```python
from build123d import *

# Parameters (mm, degrees)
F1_DEPTH = 26
F2_R     = 1
F3_SIZE  = 1
F5_DEPTH = 6.5


with BuildPart() as f1:
    # F0 (on Front) → F1 (new body)
    with BuildSketch(Plane.XZ):
        Polygon((-27.5, -55), (-20.5, -55), (27.5, -36.5), (27.5, -26.5), (-17.5, -26.5), (-17.5, 26.5), (27.5, 26.5), (27.5, 36.5), (-20.5, 55), (-27.5, 55), (-27.5, 22.5), (-24, 22.5), (-24, -22.5), (-27.5, -22.5), align=None)
        Polygon((-20.5, -31.5), (26.5698068675, -31.5), (-20.5, -49.6414880635), align=None, mode=Mode.SUBTRACT)
        Polygon((-20.5, 31.5), (-20.5, 49.6414880635), (26.5698068675, 31.5), align=None, mode=Mode.SUBTRACT)
    extrude(amount=F1_DEPTH)

    # F2
    f2_edges = [f1.edges().sort_by_distance(p)[0] for p in [
        (-20.5, -13, 49.641488),
        (-20.5, -13, 31.5),
        (26.569807, -13, 31.5),
        (26.569807, -13, -31.5),
        (-20.5, -13, -31.5),
        (-20.5, -13, -49.641488),
        (-24, -13, -22.5),
        (-24, -13, 22.5),
    ]]
    fillet(f2_edges, radius=F2_R)

    # F3
    f3_edges = [f1.edges().sort_by_distance(p)[0] for p in [
        (27.5, -13, -26.5),
        (27.5, -13, 26.5),
    ]]
    chamfer(f3_edges, length=F3_SIZE)

    # F4 (on face) → F5 (cut, through all)
    with BuildSketch(Plane.YZ.offset(-17.5)):
        with BuildLine():
            ThreePointArc((-9.25, 8), (-9.8357864376, 9.4142135624), (-11.25, 10))
            Line((-11.25, 10), (-14.75, 10))
            ThreePointArc((-14.75, 10), (-16.1642135624, 9.4142135624), (-16.75, 8))
            Line((-16.75, 8), (-16.75, -8))
            ThreePointArc((-16.75, -8), (-16.1642135624, -9.4142135624), (-14.75, -10))
            Line((-14.75, -10), (-11.25, -10))
            ThreePointArc((-11.25, -10), (-9.8357864376, -9.4142135624), (-9.25, -8))
            Line((-9.25, -8), (-9.25, 8))
        make_face()
    extrude(amount=-F5_DEPTH, mode=Mode.SUBTRACT)


solid = f1.part
```
Here's how the part is built. I have some questions about the finished solid (model axes, mm). A direction names the side the tool comes from. Coordinates: 2 decimals unless noted, no trailing zeros. Write each loop counter-clockwise with the first axis right and the second up, starting at its lowest first coordinate (ties: lowest second). Pieces come first, ordered by that corner, then holes. Notation, with made-up numbers: (54, -32) - (102, -32) arc R22 cw to (102, -18) - close; hole circle Ø5 at (-18.75, 55). An arc over 180 degrees is marked (long way). One line per item, written item: value.
1) Suppose I cut it at A-A on x = -22. Write out the boundary of the cut face in (y, z).
Model answer:
outline: (-26, -55) - (0, -55) - (0, 55) - (-26, 55) - close; hole (-16.75, -8) arc R2 ccw to (-14.75, -10) - (-11.25, -10) arc R2 ccw to (-9.25, -8) - (-9.25, 8) arc R2 ccw to (-11.25, 10) - (-14.75, 10) arc R2 ccw to (-16.75, 8) - close
2) I need wall thicknesses on line 1 along Z through (x, y) = (-2.5, -22.5); line 2 along Z through (x, y) = (7.5, -1.5); line 3 along X through (y, z) = (-7, -3.5). Which ranges of each line are inside material? Lowest first, please.
Model answer:
line 1: z = -48.06 to -42.7, -31.5 to -26.5, 26.5 to 31.5, 42.7 to 48.06
line 2: z = -44.21 to -38.85, -31.5 to -26.5, 26.5 to 31.5, 38.85 to 44.21
line 3: x = -24 to -17.5
3) Suppose I cut it at B-B on z = -6. Write out the boundary of the cut face in (x, y).
Model answer:
outline: (-24, -26) - (-17.5, -26) - (-17.5, -16.75) - (-24, -16.75) - close; (-24, -9.25) - (-17.5, -9.25) - (-17.5, 0) - (-24, 0) - close
4) Suppose I cut it at C-C on y = -21.25. State how many separate pieces and enclosed holes the cut face has, and give its area (3 significant figures).
Model answer:
separate pieces: 1
enclosed holes: 2
area: 1,770 mm²
5) On a 3-axis mill with a long thin cutter (end or side, diameter ignored), from which of +Z, -Z, +X, -X, +Y, -Y can I reach the whole of each face in a straight line? I mean faces 1 (the flat face through (-17.5, -7, 0)), 2 (the flat face through (27.5, -13, -32)), 3 (the cylindrical face through (-20.7, -16.15, 9.43)), 4 (the flat face through (-26, -13, 22.5)), 5 (the flat face through (1, -13, 31.5)). Say none if no direction works.
Model answer:
face 1: +X, +Y, -Y
face 2: +Z, -Z, +X, +Y, -Y
face 3: +X, -X
face 4: -X, +Y, -Y
face 5: +Y, -Y
6) I'm going to push flat-ended pins straight in: P1, Ø8, axis at x = 7, y = -7.5, coming from the -Z side; P2, Ø2, axis at x = 15.5, y = -11, coming from the +Z side; P3, Ø5, axis at y = -18, z = 4, coming from the +X side. Where does each tip first touch, or does it pass through?
Model answer:
P1: stops at z = -45.94
P2: stops at z = 41.51
P3: stops at x = -17.5
7) Suppose I cut it at D-D on x = 24.5. Write out the boundary of the cut face in (y, z).
Model answer:
outline: (-26, -37.66) - (0, -37.66) - (0, -26.5) - (-26, -26.5) - close; (-26, 26.5) - (0, 26.5) - (0, 37.66) - (-26, 37.66) - close
8) We'd pull the mould along Z, two halves only. Please class faces 6 (the flat face through (5, -13, -26.5)), 7 (the flat face through (3.84, -12.82, 45.62)), 8 (the flat face through (3.16, -12.82, -45.88)): pulls with the +Z half, pulls with the -Z half, needs draft (parallel to the pull), parting line crosses it, or undercut.
Model answer:
face 6: undercut
face 7: pulls with the +Z half
face 8: pulls with the -Z half
